For this review, take the finished solid that the model builds, in its own axes (mm). A direction names the side the tool comes from. Round coordinates to 2 decimals unless told otherwise and drop trailing zeros. Write each loop counter-clockwise with the first axis right and the second up, starting at its lowest first coordinate (ties: lowest second). Pieces come first, ordered by that corner, then holes. Notation, with made-up numbers: M -27,59.5 L 18,59.5 A23 cw 18,84.5 Z; hole C 15.5,73.5 d10. An arc over 180 degrees is marked long. Write each question's results on one line, items separated by ' | '. Start each with the question number.
```python
from build123d import *

# Parameters (mm, degrees)
F0_W     = 38.1
F0_H     = 63.5
F0_R     = 2.54
F0_W_2   = 25.4
F0_H_2   = 25.4
F1_DEPTH = 25.4
F2_R     = 5.08


with BuildPart() as f1:
    # F0 (on Top) → F1 (new body)
    with BuildSketch(Plane.XY):
        with Locations((-19.05, 31.75)):
            Rectangle(F0_W, F0_H)
        with Locations((-20.244129, 16.207738)):
            Circle(F0_R, mode=Mode.SUBTRACT)
        with Locations((-20.244129, 46.541594)):
            Circle(F0_R, mode=Mode.SUBTRACT)
        with Locations((12.7, -12.7)):
            Rectangle(F0_W_2, F0_H_2)
        with BuildLine():
            Line((0, -25.4), (0, 0))
            Line((0, 0), (-38.1, 0))
            add(Edge.make_bspline(
                [(-38.1, 0), (-37.680859, -22.843237), (-24.310233, -25.4), (0, -25.4)],
                knots=[0, 0, 0, 0, 45.790501, 45.790501, 45.790501, 45.790501], degree=3))
        make_face()
    extrude(amount=F1_DEPTH)

    # F2
    f2_edges = [f1.edges().sort_by_distance(p)[0] for p in [
        (-38.1, 31.75, 25.4),
        (-38.1, 31.75, 0),
        (-26.310812, -22.093817, 25.4),
        (-26.310812, -22.093817, 0),
    ]]
    fillet(f2_edges, radius=F2_R)


solid = f1.part
```
Item 1: For probe 1 along Y at (x, z) = (4.5, 14); probe 2 along X at (y, z) = (48, 14); probe 3 along X at (y, z) = (42, 13.5), list the stretches that pass through material, from the lowest coordinate up.
Item 2: For faces 5 (the flat face through (-19, 63.5, 13)), 6 (the flat face through (0, 31, 13)), list the 3-axis set-ups (+Z, -Z, +X, -X, +Y, -Y) from which the entire face can be reached by the end or side of a thin tool; tool diameter is ignored.
Item 3: Mouldability with a two-part tool opening along X and no side actions: class faces 1 (the flat face through (-38.1, 31, 13)), 2 (the flat face through (25.4, -13, 13)), 3 (the cylindrical face through (-18.879, 48.683, 12.522)), 4 (the cylindrical face through (12.522, -23.951, 23.872)) as pulls with the +X half, pulls with the -X half, needs draft (parallel to the pull), parting line crosses it, or undercut.
Item 4: Insertion check: P1, Ø4, axis at x = -6.5, z = 12, coming from the -Y side; P2, Ø4.5, axis at x = -20.24, y = 16.21, coming from the +Z side; P3, Ø12.5, axis at x = 6.5, z = 11.5, coming from the +Y side; P4, Ø2, axis at y = 42, z = 14.5, coming from the +X side. Each pin has a flat end and moves straight along its axis. Give the tip position at first contact, or say it passes through.
Item 5: We need section B-B on x = -21.5. State how many separate pieces and enclosed holes the cut face has, then the cut area to 3 significant figures.
Item 6: We need section A-A on y = 33.5. State the section outline as (x, z) points.
Numbers:
1) probe 1: y = -25.4 to 0 | probe 2: x = -38.1 to -22.32, -18.16 to 0 | probe 3: x = -38.1 to 0
2) face 5: +Z, -Z, +X, -X, +Y | face 6: +Z, -Z, +X, +Y
3) face 1: pulls with the -X half | face 2: pulls with the +X half | face 3: undercut | face 4: needs draft
4) P1: stops at y = -25.36 | P2: passes through | P3: stops at y = 0 | P4: stops at x = 0
5) separate pieces: 3 | enclosed holes: 0 | area: 1,980 mm^2
6) outline: M -38.1,5.08 A5.08 ccw -33.02,0 L 0,0 L 0,25.4 L -33.02,25.4 A5.08 ccw -38.1,20.32 Z
